from build123d import *

# Parameters (mm, degrees)
F0_R     = 2
F1_DEPTH = 3


with BuildPart() as f1:
    # F0 (on Front) → F1 (new body)
    with BuildSketch(Plane.XZ):
        with BuildLine():
            Line((27.974745, 5.446434), (3.460605, 2.876493))
            ThreePointArc((3.460605, 2.876493), (4.232182, 1.529261), (4.5, 0))
            ThreePointArc((4.5, 0), (4.191191, -1.638267), (3.307147, -3.051685))
            Line((3.307147, -3.051685), (27.655492, -6.886493))
            ThreePointArc((27.655492, -6.886493), (28.490456, -0.737511), (27.974745, 5.446434))
        make_face()
        with Locations((25.262442, -3.472612)):
            Circle(F0_R, mode=Mode.SUBTRACT)
        with BuildLine():
            ThreePointArc((-0.260659, 2.486374), (1.673074, 1.857639), (2.5, 0))
            ThreePointArc((2.5, 0), (1.624442, -1.900312), (-0.38895, -2.469558))
            Line((-0.38895, -2.469558), (3.307147, -3.051685))
            ThreePointArc((3.307147, -3.051685), (4.191191, -1.638267), (4.5, 0))
            ThreePointArc((4.5, 0), (4.232182, 1.529261), (3.460605, 2.876493))
            Line((3.460605, 2.876493), (-0.260659, 2.486374))
        make_face()
        with BuildLine():
            ThreePointArc((-0.38895, -2.469558), (-2.499163, 0.064694), (-0.260659, 2.486374))
            Line((-0.260659, 2.486374), (3.460605, 2.876493))
            ThreePointArc((3.460605, 2.876493), (-4.498493, 0.116449), (3.307147, -3.051685))
            Line((3.307147, -3.051685), (-0.38895, -2.469558))
        make_face()
    extrude(amount=F1_DEPTH)


solid = f1.part
Model file for the job. Use its own axes, mm. A direction names the side the tool comes from. Coordinates: 2 decimals unless noted, no trailing zeros. Write each loop counter-clockwise with the first axis right and the second up, starting at its lowest first coordinate (ties: lowest second). Pieces come first, ordered by that corner, then holes. Notation, with made-up numbers: (-33.75, 16) - (1.25, 16) arc R20 ccw to (1.25, 46) - close; hole circle Ø4 at (76.5, 31.25). An arc over 180 degrees is marked (long way). Write each question's results on one line, items separated by ' | '. Start each with the question number.
1) Cut at C-C (y = -0.65). Write the cut outline in (x, z), then the cut area to 3 significant figures.
2) 3-axis set-ups, long thin cutter, end or side, ignore diameter. For faces 1 (the face through (23.264, -1.479, -3.385)), 2 (the face through (15.89, -1.48, 4.18)), 3 (the face through (15.311, -1.479, -4.942)): which of +Z, -Z, +X, -X, +Y, -Y reach the whole face in a straight line?
3) Flat gauge pin, fed straight in: P1, Ø1, axis at x = -0.5, y = -1, coming from the -Z side. Where does the tip first touch, or does it go through?
4) Probe line 1 along X through (y, z) = (-2.55, 0); line 2 along X through (y, z) = (-0.2, -2); line 3 along X through (y, z) = (-1.9, 1). List the from-to ranges inside material, lowest first. Write a range as from..to.
5) Cut at B-B (x = 1.5). Write the cut outline in (y, z).
6) Cut at A-A (z = -0.75). Write the cut outline in (x, y).
7) Cut at D-D (x = 9). Write the cut outline in (y, z), then the cut area to 3 significant figures.
8) Mould opens along X. For faces 4 (the face through (28.49, -1.48, -0.82)), 5 (the face through (15, 0, -1)), 6 (the face through (-4.49, -1.48, 0.27)) say: pulls with the +X half, pulls with the -X half, needs draft (parallel to the pull), parting line crosses it, or undercut.
Returned:
1) outline: (3.31, -3.05) - (27.66, -6.89) arc R28.5 ccw to (27.97, 5.45) - (3.46, 2.88) arc R4.5 ccw (long way) to start; hole (-0.39, -2.47) arc R2.5 ccw to (2.5, 0) arc R2.5 ccw (long way) to start; hole circle Ø4 at (25.26, -3.47) | area: 256 mm^2
2) face 1: +Y, -Y | face 2: +Z, +Y, -Y | face 3: -Z, +Y, -Y
3) P1: z = -4.5
4) line 1: -4.5..-2.5, 2.5..28.5 | line 2: -4.03..-1.5, 1.5..23.91, 26.62..28.43 | line 3: -4.39..-2.29, 2.29..28.48
5) outline: (-3, -4.24) - (0, -4.24) - (0, -2) - (-3, -2) - close; (-3, 2) - (0, 2) - (0, 4.24) - (-3, 4.24) - close
6) outline: (-4.44, -3) - (-2.38, -3) - (-2.38, 0) - (-4.44, 0) - close; (2.38, -3) - (28.49, -3) - (28.49, 0) - (2.38, 0) - close
7) outline: (-3, -3.95) - (0, -3.95) - (0, 3.46) - (-3, 3.46) - close | area: 22.2 mm^2
8) face 4: pulls with the +X half | face 5: needs draft | face 6: undercut
